Check sheet for the modelled part. Datum: model origin and axes. Units: mm. Face numbers are marked on the shaded views. A direction names the side the tool comes from. Round coordinates to 2 decimals unless told otherwise and drop trailing zeros. Loops run counter-clockwise (first coordinate to the right, second up) from the corner with the lowest first, then second, coordinate; pieces in that order, holes last. Notation, with made-up numbers: (84, 13.5) - (132, 13.5) arc R25 ccw to (132, 47.5) - close; hole circle Ø9 at (76.25, -13). An arc over 180 degrees is marked (long way). Put each result on its own line as item: value.
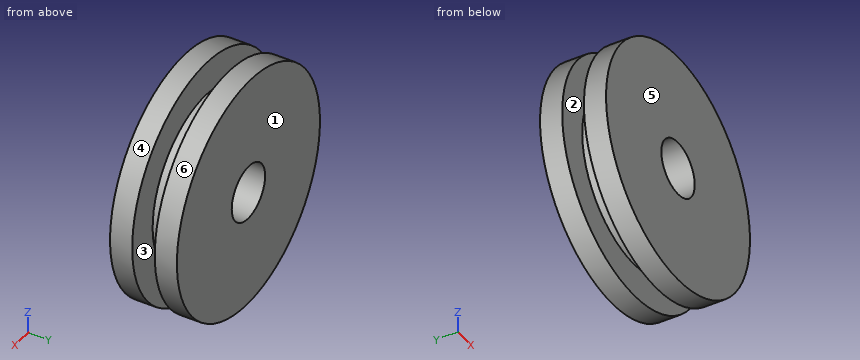
```python
from build123d import *


with BuildPart() as part:
    # Sketch1 → Revolve1 (revolve)
    with BuildSketch(Plane.YZ, mode=Mode.PRIVATE) as revolve1_sk:
        Polygon((-14.999881438, 0.027408751), (-14.999881438, 15.415581909), (-4.999994159, 15.415581909), (-4.999994159, 0.109652172), (5.000005829, 0.109652172), (5.000005829, 15.109652172), (15.000005829, 15.109652172), (15.000005829, 0.109652172), (15.000005829, -25.956139131), (-14.999881438, -25.956139131), align=None)
    revolve(revolve1_sk.sketch.rotate(Axis((0, -15, -38.456139131), (0, 1, 0)), 180), axis=Axis((0, -15, -38.456139131), (0, 1, 0)))


solid = part.part
```
Item 1: Release check for a two-part mould opening along Y. For the marked faces 1, 2, 3 and 4 record: +Y half, -Y half, draft (parallel to the pull), parting line (faces both ways), or undercut.
Filled sheet:
face 1: +Y half
face 2: undercut
face 3: undercut
face 4: draft
Item 2: Go/stop test with flat-tipped pins: pin 1 (4 mm diameter, centred on y = -4, z = -16, fed in from -X); pin 2 (5 mm diameter, centred on y = -4, z = -73.5, fed in from -X); pin 3 (5 mm diameter, centred on y = 3.5, z = -80, fed in from +X); pin 4 (22.5 mm diameter, centred on x = 0, z = -38.46, fed in from +Y). Record where each tip stops, or that it passes through.
Filled sheet:
pin 1: x = -49.73
pin 2: x = -42.77
pin 3: x = 36.13
pin 4: through
Item 3: Section check A-A on x = 0. Enter the section's corners in (y, z).
Filled sheet:
outline: (-15, -92.33) - (-5, -92.33) - (-5, -77.02) - (5, -77.02) - (5, -92.02) - (15, -92.02) - (15, -50.96) - (-15, -50.96) - close; (-15, -25.96) - (15, -25.96) - (15, 15.11) - (5, 15.11) - (5, 0.11) - (-5, 0.11) - (-5, 15.42) - (-15, 15.42) - close
Item 4: Tool access check on the marked faces 5 and 6. Record the directions out of +Z, -Z, +X, -X, +Y, -Y that give a thin tool (end or side, any length) a straight path to the whole face; none if there is none.
Filled sheet:
face 5: +Z, -Z, +X, -X, -Y
face 6: +Y
Item 5: Thickness scan on line 1 (Z direction, x = 0.5, y = -12.25); line 2 (Y direction, x = -20.5, z = -77); line 3 (Z direction, x = -2, y = -11.5). Record the ranges inside material, lowest first. Write a range as from..to.
Filled sheet:
line 1: -92.33..-50.95, -25.97..15.41
line 2: -15..-5, 5..15
line 3: -92.29..-50.8, -26.12..15.38
Item 6: Section check C-C on z = -5.5. Enter the section's corners in (x, y), then the cut area to 3 significant figures.
Filled sheet:
outline: (-42.62, -15) - (42.62, -15) - (42.62, -5) - (20.03, -5) - (20.03, 5) - (42.23, 5) - (42.23, 15) - (-42.23, 15) - (-42.23, 5) - (-20.03, 5) - (-20.03, -5) - (-42.62, -5) - close
area: 2,100 mm²
Item 7: Section check D-D on x = -44. Enter the section's corners in (y, z), then the cut area to 3 significant figures.
Filled sheet:
outline: (-15, -69.54) - (-5, -69.54) - (-5, -7.37) - (-15, -7.37) - close; (5, -69.01) - (15, -69.01) - (15, -7.91) - (5, -7.91) - close
area: 1,230 mm²
Item 8: Section check B-B on y = 1. Enter the section's corners in (x, z).
Filled sheet:
outline: circle Ø77.13 at (0, -38.46); hole circle Ø25 at (0, -38.46)
